from build123d import *

# Parameters (mm, degrees)
SKETCH2_W           = 63.5
SKETCH2_H           = 27.94
BOSS_EXTRUDE1_DEPTH = 3.175
SKETCH3_W           = 3.175
SKETCH3_H           = 15.24
CUT_EXTRUDE1_DEPTH  = 70.447636569


with BuildPart() as part:
    # Sketch2 → Boss-Extrude1 (new body)
    with BuildSketch(Plane(origin=(0, 0, 0), x_dir=(1, 0, 0), z_dir=(0, 1, 0))):
        with Locations((31.75, 13.97)):
            Rectangle(SKETCH2_W, SKETCH2_H)
    extrude(amount=BOSS_EXTRUDE1_DEPTH)

    # Sketch3 → Cut-Extrude1 (cut, through all)
    with BuildSketch(Plane.XZ):
        with Locations((19.05, -7.62)):
            Rectangle(SKETCH3_W, SKETCH3_H)
    extrude(amount=-CUT_EXTRUDE1_DEPTH, mode=Mode.SUBTRACT)


solid = part.part
The listing builds one solid part. Answer for the finished solid, in the listing's coordinates (mm). A direction names the side the tool comes from. Coordinates: 2 decimals unless noted, no trailing zeros. Loops run counter-clockwise (first coordinate to the right, second up) from the corner with the lowest first, then second, coordinate; pieces in that order, holes last. Notation, with made-up numbers: M 3.5,-31 L 27.5,-31 A15 ccw 27.5,-11 Z; hole C -24.5,55.25 d6. An arc over 180 degrees is marked long. Answer in a Markdown table with one row per item.
1) Given pin 1 (1 mm diameter, centred on x = 19, y = 1, fed in from +Z), flat-ended and moving along its own axis, determine where the tip first touches the part or whether it passes through.
Answers below:
| item | result |
|---|---|
| pin 1 | z = -15.24 |
2) Find the intervals of material crossed by probe 1 along X at (y, z) = (2.4, -9), in increasing order.
Answers below:
| item | result |
|---|---|
| probe 1 | 0 to 17.46, 20.64 to 63.5 |
3) Determine the mould class of faces 1 (the flat face through (0, 2, -14)), 2 (the flat face through (17.463, 2, -8)), 3 (the flat face through (63.5, 2, -14)), 4 (the flat face through (31, 2, -27.94)) for opening direction X: released by +X, released by -X, zero draft, split by the parting line, or undercut.
Answers below:
| item | result |
|---|---|
| face 1 | released by -X |
| face 2 | undercut |
| face 3 | released by +X |
| face 4 | zero draft |
4) Find section A-A (z = -2.75). Determine the outline of the cut face in (x, y) (1 decimal).
Answers below:
| item | result |
|---|---|
| outline | M 0,0 L 17.5,0 L 17.5,3.2 L 0,3.2 Z; M 20.6,0 L 63.5,0 L 63.5,3.2 L 20.6,3.2 Z |
5) Which of the six approach directions +Z, -Z, +X, -X, +Y, -Y give full straight-line access (tool end or side, diameter ignored) to faces 5 (the flat face through (9, 2, 0)), 6 (the flat face through (20.638, 2, -8))?
Answers below:
| item | result |
|---|---|
| face 5 | +Z, +X, -X, +Y, -Y |
| face 6 | +Z, +Y, -Y |
6) Find section B-B (y = 2.55). Determine the outline of the cut face in (x, z).
Answers below:
| item | result |
|---|---|
| outline | M 0,-27.94 L 63.5,-27.94 L 63.5,0 L 20.64,0 L 20.64,-15.24 L 17.46,-15.24 L 17.46,0 L 0,0 Z |
